The listing builds one solid part. Answer for the finished solid, in the listing's coordinates (mm). A direction names the side the tool comes from. Give positions to 0.01 mm unless a question says otherwise; leave off trailing zeros. Order: outer loops, then holes, each group sorted by start corner. A loop starts at its lowest first (then second) coordinate and runs counter-clockwise, first axis right, second up.
```python
from build123d import *

# Parameters (mm, degrees)
F0_R        = 38.6786134899
F0_R_2      = 20.6427828865
F1_DEPTH    = 12.7
F2_T        = -2.54
F3_T4_DEPTH = 240.9522929605
F3_S5_R     = 41.5273672124
F3_T6_DEPTH = 123


# Not quite as in the source:
# - a fillet or chamfer that OpenCascade refuses, or shapes differently, is made with other operations: its cross-section is extruded or revolved along the edge and cut away or added


with BuildPart() as f1:
    # F0 (on Front) → F1 (new body)
    with BuildSketch(Plane.XZ):
        with BuildLine():
            ThreePointArc((-94.9406012258, -72.3378666508), (-50.4602870277, -47.6856781771), (-32.7881381913, 0))
            ThreePointArc((-32.7881381913, 0), (-47.5673995621, 44.0958373502), (-85.9349974728, 70.3788521857))
            ThreePointArc((-85.9349974728, 70.3788521857), (-178.9877879079, 4.6081079803), (-94.9406012258, -72.3378666508))
        make_face()
        with Locations((-105.9605851769, 0)):
            Circle(F0_R, mode=Mode.SUBTRACT)
        with BuildLine():
            ThreePointArc((-85.9349974728, 70.3788521857), (-47.5673995621, 44.0958373502), (-32.7881381913, 0))
            ThreePointArc((-32.7881381913, 0), (-50.4602870277, -47.6856781771), (-94.9406012258, -72.3378666508))
            Line((-94.9406012258, -72.3378666508), (57.8033803815, -49.0687780824))
            ThreePointArc((57.8033803815, -49.0687780824), (10.4955177286, -14.2692006943), (45.2950951166, 33.0386619586))
            Line((45.2950951166, 33.0386619586), (-85.9349974728, 70.3788521857))
        make_face()
        with BuildLine():
            ThreePointArc((93.0766049614, -8.0150580619), (78.6121658048, 23.4828808015), (45.2950951166, 33.0386619586))
            ThreePointArc((45.2950951166, 33.0386619586), (10.4955177286, -14.2692006943), (57.8033803815, -49.0687780824))
            ThreePointArc((57.8033803815, -49.0687780824), (83.0471766125, -35.0779861176), (93.0766049614, -8.0150580619))
        make_face()
        with Locations((51.5492377491, -8.0150580619)):
            Circle(F0_R_2, mode=Mode.SUBTRACT)
    extrude(amount=F1_DEPTH)

    # F2
    f2_openings = [f1.faces().sort_by_distance(p)[0] for p in [
        (-50.29361, -12.7, -3.378795),
    ]]
    offset(amount=F2_T, openings=f2_openings, kind=Kind.INTERSECTION)

    # F3: chamfer of 5.08 on 1 edges, made by hand


with BuildPart() as f3_tool2:
    # F3_s3 → F3_t4 (new body)
    with BuildSketch(Plane(origin=(96.0327547633, 0, -27.3251451716), x_dir=(0, 1, 0), z_dir=(-0.961821766, 0, 0.2736766164))):
        Polygon((-7.62, -44.1735125635), (-12.7, -39.0935125635), (-12.7, -44.1735125635), align=None)
    extrude(amount=F3_T4_DEPTH)

    # F3_s5 → F3_t6 (cut, symmetric)
    with BuildSketch(Plane.XZ.offset(10.2)):
        with Locations((51.5492377491, -8.0150580619)):
            Circle(F3_S5_R)
    extrude(amount=F3_T6_DEPTH, both=True, mode=Mode.SUBTRACT)


with BuildPart() as f1_1:
    add(f1.part)

    # F3_t1: cut F3_tool2
    add(f3_tool2.part, mode=Mode.SUBTRACT)


solid = f1_1.part
```
1) Find section C-C (x = -73). Write down the section's boundary in (y, z).
Geometry says:
outline: (-12.7, -69) - (0, -69) - (0, -20.24) - (-12.7, -20.24) - (-12.7, -24.75) - (-2.54, -24.75) - (-2.54, -66.43) - (-12.7, -66.43) - close; (-12.7, 20.24) - (0, 20.24) - (0, 66.7) - (-7.62, 66.7) - (-10.16, 64.06) - (-2.54, 64.06) - (-2.54, 24.75) - (-12.7, 24.75) - close
2) Find section B-B (z = -5). Write down the section's boundary in (x, y), then the cut area to 3 significant figures.
Geometry says:
outline: (-178.96, -12.7) - (-176.42, -12.7) - (-176.42, -2.54) - (-146.87, -2.54) - (-146.87, -12.7) - (-144.31, -12.7) - (-144.31, 0) - (-178.96, 0) - close; (-67.61, -12.7) - (-65.05, -12.7) - (-65.05, -2.54) - (28.56, -2.54) - (28.56, -12.7) - (31.13, -12.7) - (31.13, 0) - (-67.61, 0) - close; (71.97, -12.7) - (74.54, -12.7) - (74.54, -2.54) - (90.42, -2.54) - (90.42, -12.7) - (92.97, -12.7) - (92.97, 0) - (71.97, 0) - close
area: 548 mm2
3) Find section A-A (y = -5.5). Write down the section's boundary in (x, z) (3 decimals).
Geometry says:
outline: circle Ø82.437 at (-105.961, 0); (-94.941, -72.338) - (57.803, -49.069) arc R41.527 ccw to (45.295, 33.039) - (-85.935, 70.379) arc R73.172 ccw (long way) to start; circle Ø46.366 at (51.549, -8.015); hole circle Ø77.357 at (-105.961, 0); hole (-95.323, -69.827) - (57.421, -46.558) arc R38.987 ccw (long way) to (45.14, 30.442) - (-86.63, 67.936) arc R70.632 ccw (long way) to start; hole circle Ø41.286 at (51.549, -8.015)
4) For a pull along Z with two mould halves and no side action, classify faces 1 (the cylindrical face through (-136.65, -6.26, -23.54)), 2 (the cylindrical face through (-178.85, -6.26, 6.43)), 3 (the flat face through (-54, -12.7, -65)), 4 (the flat face through (-32.48, -8.996, 53.739)) as +Z half, -Z half, draft (parallel to the pull), parting line (faces both ways), or undercut.
Geometry says:
face 1: undercut
face 2: parting line
face 3: draft
face 4: +Z half
5) A tool of negligible diameter and unlimited length cuts with its end or side. For faces 5 (the flat face through (-19.638, -6.261, -60.866)), 6 (the flat face through (-19.823, -6.42, 48.926)), from which of +Z, -Z, +X, -X, +Y, -Y can it reach the whole face along a straight path? Write none if from no direction.
Geometry says:
face 5: -Z, +X, +Y, -Y
face 6: -Y
6) Straight lines are drawn through the part: probe 1 along X at (y, z) = (-0.5, -8); probe 2 along Z at (x, y) = (-129.5, -10); probe 3 along X at (y, z) = (-11, -16) (3 decimals). For each, find the intervals that lie inside material, in ascending order.
Geometry says:
probe 1: x = -178.69 to -143.8, -68.12 to 30.91, 72.19 to 93.08
probe 2: z = -69.28 to -66.59, -33.84 to -30.69, 30.69 to 33.84, 66.59 to 69.28
probe 3: x = -177.362 to -174.757, -143.947 to -141.175, -70.746 to -67.974, 29.785 to 32.513, 70.585 to 73.313, 89.71 to 92.302
7) Given P1, Ø6, axis at x = -32.5, y = -10, coming from the +Z side; P2, Ø1, axis at y = -4, z = 22.5, coming from the -X side; P3, Ø5, axis at x = -38.5, y = -2.5, coming from the +Z side, each flat-ended and moving along its own axis, determine where each tip first touches the part or whether it passes through.
Geometry says:
P1: stops at z = 55.69
P2: stops at x = -175.75
P3: stops at z = 57.59
